Read the model definition and answer for the solid it produces. Units are mm, in the model's axes. A direction names the side the tool comes from. Give positions to 0.01 mm unless a question says otherwise; leave off trailing zeros. Order: outer loops, then holes, each group sorted by start corner. A loop starts at its lowest first (then second) coordinate and runs counter-clockwise, first axis right, second up.
```python
from build123d import *

# Parameters (mm, degrees)
SKETCH3_W           = 41.148121512
SKETCH3_H           = 40.81
SKETCH3_R           = 0.8508
BOSS_EXTRUDE1_DEPTH = 1.6
SKETCH4_W           = 9
SKETCH4_H           = 14.6
BOSS_EXTRUDE2_DEPTH = 11
SKETCH5_R           = 1.871357829
SKETCH5_R_2         = 0.869870556
CUT_EXTRUDE1_DEPTH  = 11
SKETCH6_W           = 20.324920815
SKETCH6_H           = 30.484920815
BOSS_EXTRUDE3_DEPTH = 15
SKETCH7_W           = 7.620985393
SKETCH7_H           = 2.54
SKETCH7_W_2         = 7.620835906
BOSS_EXTRUDE4_DEPTH = 9
SKETCH8_W           = 10.16
SKETCH8_H           = 40
BOSS_EXTRUDE5_DEPTH = 15


with BuildPart() as part:
    # Sketch3 → Boss-Extrude1 (new body)
    with BuildSketch(Plane(origin=(0, 0, 0), x_dir=(1, 0, 0), z_dir=(0, 1, 0))):
        with Locations((35.374060756, 20.505)):
            Rectangle(SKETCH3_W, SKETCH3_H)
        with Locations(Location((18.2, 3.5, 0), (0, 0, 270))):
            Circle(SKETCH3_R, mode=Mode.SUBTRACT)
        with Locations(Location((52.5, 37.5, 0), (0, 0, 270))):
            Circle(SKETCH3_R, mode=Mode.SUBTRACT)
        with Locations(Location((18.2, 37.5, 0), (0, 0, 270))):
            Circle(SKETCH3_R, mode=Mode.SUBTRACT)
    extrude(amount=BOSS_EXTRUDE1_DEPTH)

    # Sketch4 → Boss-Extrude2 (add)
    with BuildSketch(Plane(origin=(0, 1.6, 0), x_dir=(1, 0, 0), z_dir=(0, 1, 0))):
        with Locations((26.028, 2.965)):
            Rectangle(SKETCH4_W, SKETCH4_H)
    extrude(amount=BOSS_EXTRUDE2_DEPTH)

    # Sketch5 → Cut-Extrude1 (cut)
    with BuildSketch(Plane.XY.offset(4.335)):
        with Locations((25.972613511, 9.593081392)):
            Circle(SKETCH5_R)
        with Locations((25.972613511, 9.593081392)):
            Circle(SKETCH5_R_2, mode=Mode.SUBTRACT)
    extrude(amount=-CUT_EXTRUDE1_DEPTH, mode=Mode.SUBTRACT)

    # Sketch6 → Boss-Extrude3 (add)
    with BuildSketch(Plane(origin=(0, 1.6, 0), x_dir=(1, 0, 0), z_dir=(0, 1, 0))):
        with Locations((43.720460407, 16.687539593)):
            Rectangle(SKETCH6_W, SKETCH6_H)
    extrude(amount=BOSS_EXTRUDE3_DEPTH)

    # Sketch7 → Boss-Extrude4 (add)
    with BuildSketch(Plane(origin=(0, 1.6, 0), x_dir=(1, 0, 0), z_dir=(0, 1, 0))):
        with Locations((32.968492697, 37.275)):
            Rectangle(SKETCH7_W, SKETCH7_H)
        with Locations((42.088417953, 37.275)):
            Rectangle(SKETCH7_W_2, SKETCH7_H)
    extrude(amount=BOSS_EXTRUDE4_DEPTH)

    # Sketch8 → Boss-Extrude5 (add)
    with BuildSketch(Plane(origin=(0, 1.6, 0), x_dir=(1, 0, 0), z_dir=(0, 1, 0))):
        with Locations((21.303, 34.17)):
            Rectangle(SKETCH8_W, SKETCH8_H)
    extrude(amount=BOSS_EXTRUDE5_DEPTH)


solid = part.part
```
1) The part is cut by section A-A on x = 52.5. Determine the outline of the cut face in (y, z), and give its area (3 significant figures).
Final values:
outline: (0, -40.91) - (1.6, -40.91) - (1.6, -38.35) - (0, -38.35) - close; (0, -36.65) - (1.6, -36.65) - (1.6, -31.93) - (16.6, -31.93) - (16.6, -1.45) - (1.6, -1.45) - (1.6, -0.1) - (0, -0.1) - close
area: 520 mm2
2) The part is cut by section D-D on z = -3.5. Determine the outline of the cut face in (x, y).
Final values:
outline: (14.8, 0) - (17.35, 0) - (17.35, 1.6) - (14.8, 1.6) - close; (19.05, 0) - (55.95, 0) - (55.95, 1.6) - (53.88, 1.6) - (53.88, 16.6) - (33.56, 16.6) - (33.56, 1.6) - (30.53, 1.6) - (30.53, 12.6) - (21.53, 12.6) - (21.53, 1.6) - (19.05, 1.6) - close; circle Ø1.74 at (25.97, 9.59); hole circle Ø3.74 at (25.97, 9.59)
3) For a pull along Z with two mould halves and no side action, classify faces 4 (the face through (35, 0, -21)), 5 (the face through (44, 9, -1.445)), 6 (the face through (21, 9, -14.17)) as released by +Z, released by -Z, zero draft, split by the parting line, or undercut.
Final values:
face 4: zero draft
face 5: released by +Z
face 6: undercut
4) Consider L1, parallel to X at y = 1.25, z = -37.5; L2, parallel to X at y = 2, z = -28; L3, parallel to Z at x = 44.5, y = 6.75 (3 decimals). Determine where each line is inside the solid, lowest interval first.
Final values:
L1: x = 14.8 to 17.35, 19.05 to 51.65, 53.35 to 55.95
L2: x = 16.22 to 26.38, 33.56 to 53.88
L3: z = -38.545 to -36.005, -31.93 to -1.445
5) The part is cut by section B-B on z = -37.5. Determine the outline of the cut face in (x, y), and give its area (3 significant figures).
Final values:
outline: (14.8, 0) - (17.35, 0) - (17.35, 1.6) - (19.05, 1.6) - (19.05, 0) - (51.65, 0) - (51.65, 1.6) - (45.9, 1.6) - (45.9, 10.6) - (38.28, 10.6) - (38.28, 1.6) - (36.78, 1.6) - (36.78, 10.6) - (29.16, 10.6) - (29.16, 1.6) - (26.38, 1.6) - (26.38, 16.6) - (16.22, 16.6) - (16.22, 1.6) - (14.8, 1.6) - close; (53.35, 0) - (55.95, 0) - (55.95, 1.6) - (53.35, 1.6) - close
area: 350 mm2
6) A tool of negligible diameter and unlimited length cuts with its end or side. For faces 1 (the face through (18, 1.6, -38)), 2 (the face through (33, 10.6, -37)), 3 (the face through (16.223, 9, -34)), from which of +Z, -Z, +X, -X, +Y, -Y can it reach the whole face along a straight path? Write none if from no direction.
Final values:
face 1: -Y
face 2: -Z, +X, +Y
face 3: +Z, -Z, -X, +Y
7) The part is cut by section C-C on y = 6. Determine the outline of the cut face in (x, z) (3 decimals).
Final values:
outline: (16.223, -54.17) - (26.383, -54.17) - (26.383, -14.17) - (16.223, -14.17) - close; (21.528, -10.265) - (30.528, -10.265) - (30.528, 4.335) - (21.528, 4.335) - close; (29.158, -38.545) - (36.779, -38.545) - (36.779, -36.005) - (29.158, -36.005) - close; (33.558, -31.93) - (53.883, -31.93) - (53.883, -1.445) - (33.558, -1.445) - close; (38.278, -38.545) - (45.899, -38.545) - (45.899, -36.005) - (38.278, -36.005) - close
8) Given pin 1 (3 mm diameter, centred on y = 9, z = -29, fed in from +X); pin 2 (3.5 mm diameter, centred on y = 7, z = -1, fed in from -X); pin 3 (4 mm diameter, centred on x = 41.5, y = 8.5, fed in from +Z), each flat-ended and moving along its own axis, determine where each tip first touches the part or whether it passes through.
Final values:
pin 1: stops at x = 53.88
pin 2: stops at x = 21.53
pin 3: stops at z = -1.45
